from build123d import *

# Parameters (mm, degrees)
BOSS_EXTRUDE1_DEPTH = 25.4
BOSS_EXTRUDE2_DEPTH = 215.9
SKETCH3_R           = 10.795
CUT_EXTRUDE1_DEPTH  = 381


with BuildPart() as part:
    # Sketch1 → Boss-Extrude1 (new body)
    with BuildSketch(Plane(origin=(0, 0, 0), x_dir=(1, 0, 0), z_dir=(0, 1, 0))):
        Polygon((0, 0), (148.510590519, -34.210590519), (34.210590519, 148.510590519), align=None)
    extrude(amount=BOSS_EXTRUDE1_DEPTH)

    # Sketch2 → Boss-Extrude2 (add)
    with BuildSketch(Plane(origin=(0, 25.4, 0), x_dir=(1, 0, 0), z_dir=(0, 1, 0))):
        Polygon((34.210590519, 148.510590519), (22.983547144, 99.773202004), (99.773202004, -22.983547144), (148.510590519, -34.210590519), align=None)
    extrude(amount=-BOSS_EXTRUDE2_DEPTH)

    # Sketch3 → Cut-Extrude1 (cut)
    with BuildSketch(Plane(origin=(61.378374574, 0, -38.39482743), x_dir=(0.5303300858898913, 0, 0.8477912478906706), z_dir=(-0.8477912478906706, 0, 0.5303300858898913))):
        with Locations((0, -38.1)):
            Circle(SKETCH3_R)
        with Locations((0, -114.3)):
            Circle(SKETCH3_R)
        with Locations((0, -152.4)):
            Circle(SKETCH3_R)
        with Locations((0, -76.2)):
            Circle(SKETCH3_R)
    extrude(amount=-CUT_EXTRUDE1_DEPTH, mode=Mode.SUBTRACT)


solid = part.part
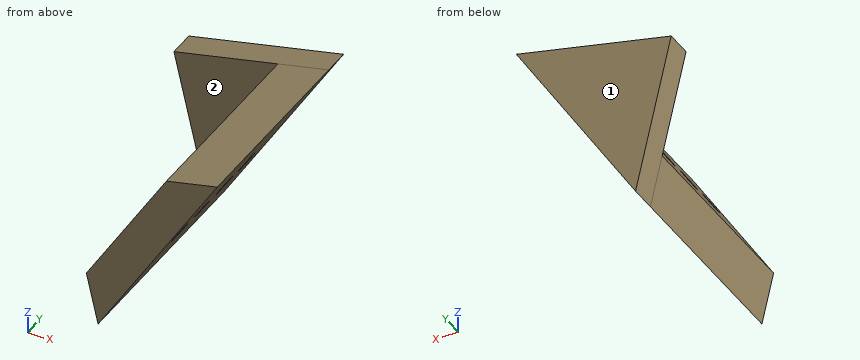
Can you work these out from the model? Positions are in its coordinate system, mm. Face numbers are marked on the shaded views. A direction names the side the tool comes from. Round coordinates to 2 decimals unless told otherwise and drop trailing zeros. Order: outer loops, then holes, each group sorted by start corner. A loop starts at its lowest first (then second) coordinate and runs counter-clockwise, first axis right, second up. Notation, with made-up numbers: (48.5, -39.5) -> (60.5, -39.5) arc R12 ccw to (60.5, -23.5) -> close; hole circle Ø9 at (86.5, 63). An arc over 180 degrees is marked (long way). Write each question's results on one line, items separated by ' | '. Start each with the question number.
Item 1: If we section it at A-A, the plane y = -149: Write out the boundary of the cut face in (x, z).
Item 2: If we section it at C-C, the plane x = 77.5: State how many separate pieces and enclosed holes the cut face has, then the cut area to 3 significant figures.
Item 3: Please list where these lines run through material, in increasing order: L1, parallel to Y at x = 76.5, z = -47.5; L2, parallel to Y at x = 25.5, z = -68.5; L3, parallel to Z at x = 119.5, y = -123.
Item 4: Will these pins go through, and if not, where does the flat tip stop? pin 1 (10 mm diameter, centred on y = -119, z = -63, fed in from +X); pin 2 (10 mm diameter, centred on x = 75.5, y = -95.5, fed in from +Z); pin 3 (1.5 mm diameter, centred on y = -166, z = -29.5, fed in from -X).
Item 5: If we section it at B-B, the plane z = -105.5: Write out the boundary of the cut face in (x, y).
Item 6: Which directions (+Z, -Z, +X, -X, +Y, -Y) give clear straight access to the entire face, cutting with the end or side of a thin tool? Please do the marked faces 1 and 2.
Item 7: If we section it at D-D, the plane y = 6: Write out the boundary of the cut face in (x, z).
Results:
1) outline: (22.98, -99.77) -> (34.21, -148.51) -> (85.93, -65.84) -> (55.94, -47.08) -> close; (66.81, -29.71) -> (96.79, -48.46) -> (148.51, 34.21) -> (99.77, 22.98) -> close
2) separate pieces: 1 | enclosed holes: 4 | area: 13,400 mm2
3) L1: y = -190.5 to -163.19, -141.61 to -125.09, -103.51 to -86.99, -65.41 to -48.89, -27.31 to 25.4 | L2: y = 0 to 25.4 | L3: z = -12.17 to 27.53
4) pin 1: stops at x = 88.62 | pin 2: stops at z = -7.83 | pin 3: stops at x = 66.47
5) outline: (24.3, -190.5) -> (61.12, -190.5) -> (61.12, 25.4) -> (24.3, 25.4) -> close
6) face 1: +Z, -Z, +X, -X, +Y | face 2: +Z, -X, -Y
7) outline: (0, 0) -> (34.21, -148.51) -> (148.51, 34.21) -> close
